Geometry: final body of the model. Coordinates: model frame, mm. A direction names the side the tool comes from. Give positions to 0.01 mm unless a question says otherwise; leave off trailing zeros. Write each loop counter-clockwise with the first axis right and the second up, starting at its lowest first coordinate (ties: lowest second). Pieces come first, ordered by that corner, then holes.
Q1. Section D-D (z = 2.25). Return the cut outline in (x, y).
Q2. Mould query, pull axis X, two halves, no side actions, for faces 4 (the flat face through (8, 0, 13.3)), 5 (the flat face through (0, 8, 13.3)), 6 (the flat face through (10, -7, 7)). Classes: +X half, -X half, draft (parallel to the pull), parting line (faces both ways), or undercut.
Q3. Section A-A (z = 13.75). Return the cut outline in (x, y), plus the area to 3 significant figures.
Q4. Section B-B (y = -4). Return the cut outline in (x, z).
Q5. Reachability of faces 1 (the flat face through (0, 6, 14)), 2 (the flat face through (8, 6, 7)), 3 (the flat face through (6, -8, 7)) from +Z, -Z, +X, -X, +Y, -Y: full face, straight path, thin tool, end or side. Return the list, or none.
Q6. Line query: line 1 (X direction, y = 6.75, z = 5.5); line 2 (Z direction, x = 3.25, y = -7). Output: solid intervals per line, ascending.
Q7. Pin query (flat end, axial travel): pin 1 Ø1 at (x, z) = (-4, 6.5) entering from +Y. Return the tip coordinate at first contact, or that it passes through.
from build123d import *

# Parameters (mm, degrees)
F0_W     = 20
F0_H     = 20
F1_DEPTH = 0.6
F2_W     = 4
F2_H     = 4
F3_DEPTH = 12.7
F6_W     = 20
F6_H     = 20
F6_W_2   = 12
F6_H_2   = 12
F7_DEPTH = 1


with BuildPart() as f1:
    # F0 (on Top) → F1 (new body)
    with BuildSketch(Plane.XY):
        Rectangle(F0_W, F0_H)
    extrude(amount=F1_DEPTH)

    # F2 (on face) → F3 (join)
    with BuildSketch(Plane.XY.offset(0.6)):
        with Locations((-8, 8)):
            Rectangle(F2_W, F2_H)
    extrude(amount=F3_DEPTH)

    # F4: F1 across plane


with BuildPart() as f1_1:
    add(f1.part)
    add(f1.part.mirror(Plane.YZ))

    # F5: F1 across plane


with BuildPart() as f1_2:
    add(f1_1.part)
    add(f1_1.part.mirror(Plane.XZ))

    # F6 (on face) → F7 (join)
    with BuildSketch(Plane.XY.offset(13.3)):
        Rectangle(F6_W, F6_H)
        Rectangle(F6_W_2, F6_H_2, mode=Mode.SUBTRACT)
    extrude(amount=F7_DEPTH)


solid = f1_2.part
Computed:
1. outline: (-10, -10) - (-6, -10) - (-6, -6) - (-10, -6) - close; (-10, 6) - (-6, 6) - (-6, 10) - (-10, 10) - close; (6, -10) - (10, -10) - (10, -6) - (6, -6) - close; (6, 6) - (10, 6) - (10, 10) - (6, 10) - close
2. face 4: draft
2. face 5: undercut
2. face 6: +X half
3. outline: (-10, -10) - (10, -10) - (10, 10) - (-10, 10) - close; hole (-6, -6) - (6, -6) - (6, 6) - (-6, 6) - close
3. area: 256 mm2
4. outline: (-10, 0) - (10, 0) - (10, 0.6) - (-10, 0.6) - close; (-10, 13.3) - (-6, 13.3) - (-6, 14.3) - (-10, 14.3) - close; (6, 13.3) - (10, 13.3) - (10, 14.3) - (6, 14.3) - close
5. face 1: +Z
5. face 2: +X, -X
5. face 3: +Y, -Y
6. line 1: x = -10 to -6, 6 to 10
6. line 2: z = 0 to 0.6, 13.3 to 14.3
7. pin 1: passes through
